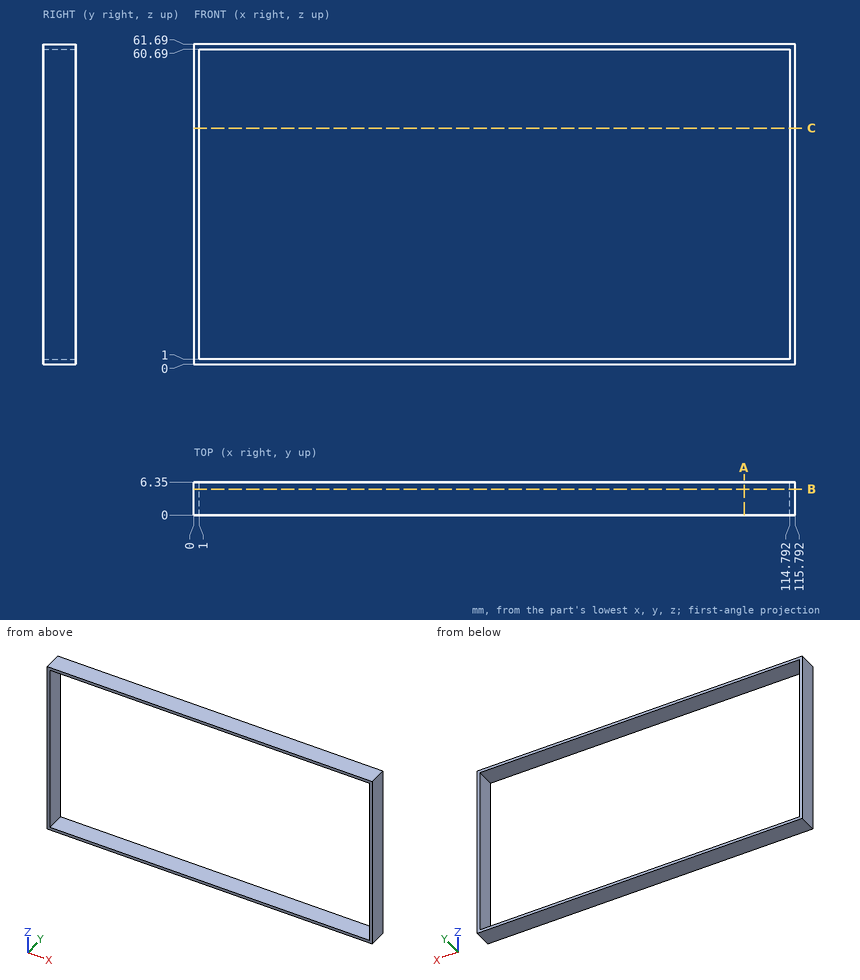
Could you check a few things on this drawing? It's one solid part, dimensions in mm from its lowest x, y, z. Give positions to 0.01 mm unless a question says otherwise; leave off trailing zeros. Write each loop counter-clockwise with the first axis right and the second up, starting at its lowest first coordinate (ties: lowest second). Pieces come first, ordered by that corner, then holes. Notation, with made-up numbers: (60.5, 16.25) -> (68.5, 16.25) arc R36 ccw to (68.5, 54.25) -> close; hole circle Ø8 at (89, -23.75). An arc over 180 degrees is marked (long way). Write item = value, one per line.
(1) Suppose I cut it at B-B on y = 5. Write out the boundary of the cut face in (x, z).
Worked out:
outline = (0, 0) -> (115.79, 0) -> (115.79, 61.69) -> (0, 61.69) -> close; hole (1, 1) -> (114.79, 1) -> (114.79, 60.69) -> (1, 60.69) -> close
(2) I need wall thicknesses on probe 1 along X at (y, z) = (2.75, 38); probe 2 along Z at (x, y) = (109, 0.75). Which ranges of each line are inside material? Lowest first, please. Write a range as from..to.
Worked out:
probe_1 = 0..1, 114.79..115.79
probe_2 = 0..1, 60.69..61.69
(3) Suppose I cut it at A-A on x = 106. Write out the boundary of the cut face in (y, z), then the cut area to 3 significant figures.
Worked out:
outline = (0, 0) -> (6.35, 0) -> (6.35, 1) -> (0, 1) -> close; (0, 60.69) -> (6.35, 60.69) -> (6.35, 61.69) -> (0, 61.69) -> close
area = 12.7 mm^2
(4) I'm going to push a flat-ended pin straight in: P1, Ø3, axis at x = 72.5, y = 4.5, coming from the -Z side. Where does the tip first touch, or does it pass through?
Worked out:
P1 = 0
(5) Suppose I cut it at C-C on z = 45.5. Write out the boundary of the cut face in (x, y).
Worked out:
outline = (0, 0) -> (1, 0) -> (1, 6.35) -> (0, 6.35) -> close; (114.79, 0) -> (115.79, 0) -> (115.79, 6.35) -> (114.79, 6.35) -> close
